Read the model definition and answer for the solid it produces. Units are mm, in the model's axes. A direction names the side the tool comes from. Coordinates: 2 decimals unless noted, no trailing zeros. Order: outer loops, then holes, each group sorted by start corner. A loop starts at its lowest first (then second) coordinate and runs counter-clockwise, first axis right, second up. Notation, with made-up numbers: (84.25, 33.5) -> (143.25, 33.5) arc R10 cw to (143.25, 50.5) -> close; hole circle Ø6 at (37.5, 79). An arc over 180 degrees is marked (long way). Return JSON: item names as keys, results as strings. Group by question number.
```python
from build123d import *

# Parameters (mm, degrees)
SKETCH_1_R      = 1.5
SKETCH_1_R_2    = 3
EXTRUDE_1_DEPTH = 0.5
SKETCH_3_R      = 1.5
SKETCH_3_R_2    = 3
EXTRUDE_2_DEPTH = 0.5
SKETCH_4_W      = 90
SKETCH_4_H      = 9
EXTRUDE_3_DEPTH = 0.5
FILLET_1_R      = 8
FILLET_2_R      = 6


with BuildPart() as part:
    # Sketch 1 → Extrude 1 (new body)
    with BuildSketch(Plane.XY):
        with BuildLine():
            Line((-28.937588447, 11.863865809), (81.062411553, 11.863865809))
            Line((81.062411553, 11.863865809), (81.062411553, 1.863865809))
            Line((81.062411553, 1.863865809), (61.338833841, 1.863865809))
            Line((61.338833841, 1.863865809), (41.922203683, -21.275972939))
            Line((41.922203683, -21.275972939), (28.562411553, 1.863865809))
            Line((28.562411553, 1.863865809), (-28.937588447, 1.863865809))
            Line((-28.937588447, 1.863865809), (-43.464520366, 0.879869346))
            ThreePointArc((-43.464520366, 0.879869346), (-50.920555651, 8.351891461), (-42.497668866, 14.714167379))
            Line((-42.497668866, 14.714167379), (-28.937588447, 11.863865809))
        make_face()
        with Locations((-43.937588447, 7.863865809)):
            Circle(SKETCH_1_R, mode=Mode.SUBTRACT)
        with Locations((42.562411553, -10.136134191)):
            Circle(SKETCH_1_R_2, mode=Mode.SUBTRACT)
        with Locations((51.562411553, -3.136134191)):
            Circle(SKETCH_1_R, mode=Mode.SUBTRACT)
        with Locations((-18.937588447, 7.863865809)):
            Circle(SKETCH_1_R, mode=Mode.SUBTRACT)
        with Locations((-8.937588447, 7.863865809)):
            Circle(SKETCH_1_R, mode=Mode.SUBTRACT)
        with Locations((62.409410938, 7.863865809)):
            Circle(SKETCH_1_R, mode=Mode.SUBTRACT)
    extrude(amount=EXTRUDE_1_DEPTH)



with BuildPart() as body_2:
    # Sketch 3 → Extrude 2 (new body)
    with BuildSketch(Plane.XY.offset(-8)):
        with BuildLine():
            Line((41.922203683, -21.275972939), (61.338833841, 1.863865809))
            Line((61.338833841, 1.863865809), (81.062411553, 1.863865809))
            Line((81.062411553, 1.863865809), (81.062411553, 11.863865809))
            Line((81.062411553, 11.863865809), (-28.937588447, 11.863865809))
            Line((-28.937588447, 11.863865809), (-42.497668866, 14.714167379))
            ThreePointArc((-42.497668866, 14.714167379), (-50.920555651, 8.351891461), (-43.464520366, 0.879869346))
            Line((-43.464520366, 0.879869346), (-28.937588447, 1.863865809))
            Line((-28.937588447, 1.863865809), (28.562411553, 1.863865809))
            Line((28.562411553, 1.863865809), (41.922203683, -21.275972939))
        make_face()
        with Locations((51.562411553, -3.136134191)):
            Circle(SKETCH_3_R, mode=Mode.SUBTRACT)
        with Locations((42.562411553, -10.136134191)):
            Circle(SKETCH_3_R_2, mode=Mode.SUBTRACT)
        with Locations((-43.937588447, 7.863865809)):
            Circle(SKETCH_3_R, mode=Mode.SUBTRACT)
        with Locations((62.409410938, 7.863865809)):
            Circle(SKETCH_3_R, mode=Mode.SUBTRACT)
        with Locations((-8.937588447, 7.863865809)):
            Circle(SKETCH_3_R, mode=Mode.SUBTRACT)
        with Locations((-18.937588447, 7.863865809)):
            Circle(SKETCH_3_R, mode=Mode.SUBTRACT)
    extrude(amount=-EXTRUDE_2_DEPTH)


with BuildPart() as part_1:
    add(part.part)

    add(body_2.part)  # Extrude 3 merges body 2
    # Sketch 4 → Extrude 3 (add)
    with BuildSketch(Plane(origin=(0, 11.863865809, 0), x_dir=(1, 0, 0), z_dir=(0, 1, 0))):
        with Locations((26.062411553, 4)):
            Rectangle(SKETCH_4_W, SKETCH_4_H)
    extrude(amount=EXTRUDE_3_DEPTH)

    # Fillet 1
    fillet_1_edges = [part_1.edges().sort_by_distance(p)[0] for p in [
        (61.338833841, 1.863865809, 0.25),
        (28.562411553, 1.863865809, 0.25),
        (28.562411553, 1.863865809, -8.25),
        (61.338833841, 1.863865809, -8.25),
    ]]
    fillet(fillet_1_edges, radius=FILLET_1_R)

    # Fillet 2
    fillet_2_edges = [part_1.edges().sort_by_distance(p)[0] for p in [
        (41.922203683, -21.275972939, 0.25),
        (41.922203683, -21.275972939, -8.25),
    ]]
    fillet(fillet_2_edges, radius=FILLET_2_R)


solid = part_1.part
```
1. Find section D-D on x = 42. Determine the outline of the cut face in (y, z).
2. Find section C-C on x = -3.5. Determine the outline of the cut face in (y, z), and give its area (3 significant figures).
3. Which of the six approach directions +Z, -Z, +X, -X, +Y, -Y give full straight-line access (tool end or side, diameter ignored) to faces 1 (the face through (25, 11.864, -4)), 2 (the face through (42.39, -16.84, 0.25)), 3 (the face through (-35.62, 13.27, -8.25))?
4. Given pin 1 (1.8 mm diameter, centred on x = 51.56, y = -3.14, fed in from +Z); pin 2 (5 mm diameter, centred on x = 20.5, z = -3.5, fed in from +Y); pin 3 (0.6 mm diameter, centred on x = -24, z = -8, fed in from +Y); pin 4 (0.6 mm diameter, centred on x = 74, z = 0, fed in from -Y), each flat-ended and moving along its own axis, determine where each tip first touches the part or whether it passes through.
5. Find section B-B on y = -12. Determine the outline of the cut face in (x, z), and give its area (3 significant figures).
6. Find section A-A on x = -23.5. Determine the outline of the cut face in (y, z), and give its area (3 significant figures).
7. Straight lines are drawn through the part: L1, parallel to Z at x = 75, y = 10.5; L2, parallel to Y at x = 3, z = -1.75; L3, parallel to X at y = -4.5, z = 0.25. For each, find the intervals that lie inside material, in ascending order.
8. For a pull along Y with two mould halves and no side action, classify faces 4 (the face through (50.372, -4.049, -8.246)), 5 (the face through (14, 6, -8)), 6 (the face through (27.893, 0.821, 0.254)) as released by +Y, released by -Y, zero draft, split by the parting line, or undercut.
Result:
{
 "1": {"outline": "(-16.8, -8.5) -> (-13.08, -8.5) -> (-13.08, -8) -> (-16.8, -8) -> close; (-16.8, 0) -> (-13.08, 0) -> (-13.08, 0.5) -> (-16.8, 0.5) -> close; (-7.19, -8.5) -> (12.36, -8.5) -> (12.36, 0.5) -> (-7.19, 0.5) -> (-7.19, 0) -> (11.86, 0) -> (11.86, -8) -> (-7.19, -8) -> close"},
 "2": {"outline": "(1.86, -8.5) -> (12.36, -8.5) -> (12.36, 0.5) -> (1.86, 0.5) -> (1.86, 0) -> (11.86, 0) -> (11.86, -8) -> (1.86, -8) -> close", "area": "14.5 mm^2"},
 "3": {"face 1": "+X, -X, -Y", "face 2": "+Z, -Z, -Y", "face 3": "+Z, -Z, +Y"},
 "4": {"pin 1": "through", "pin 2": "y = 12.36", "pin 3": "y = 11.86", "pin 4": "y = 1.86"},
 "5": {"outline": "(36.57, -8.5) -> (40.21, -8.5) -> (40.21, -8) -> (36.57, -8) -> close; (36.57, 0) -> (40.21, 0) -> (40.21, 0.5) -> (36.57, 0.5) -> close; (44.91, -8.5) -> (49.71, -8.5) -> (49.71, -8) -> (44.91, -8) -> close; (44.91, 0) -> (49.71, 0) -> (49.71, 0.5) -> (44.91, 0.5) -> close", "area": "8.44 mm^2"},
 "6": {"outline": "(1.86, -8.5) -> (11.86, -8.5) -> (11.86, -8) -> (1.86, -8) -> close; (1.86, 0) -> (11.86, 0) -> (11.86, 0.5) -> (1.86, 0.5) -> close", "area": "10.0 mm^2"},
 "7": {"L1": "-8.5 to -8, 0 to 0.5", "L2": "11.86 to 12.36", "L3": "32.24 to 50.94, 52.19 to 56"},
 "8": {"face 4": "undercut", "face 5": "zero draft", "face 6": "released by -Y"}
}
